Check sheet for the modelled part. Datum: model origin and axes. Units: mm. Face numbers are marked on the shaded views. A direction names the side the tool comes from. Round coordinates to 2 decimals unless told otherwise and drop trailing zeros. Loops run counter-clockwise (first coordinate to the right, second up) from the corner with the lowest first, then second, coordinate; pieces in that order, holes last. Notation, with made-up numbers: M 87,86 L 108,86 A23 cw 108,95 Z; hole C 64.25,-13 d4. An arc over 180 degrees is marked long. One line per question, with ' | ' between items. Start each with the question number.
(1) Section check A-A (x = 0). Record the boundary of the cut face in (y, z), and give its area (3 significant figures).
(2) Thickness scan on probe 1 along Y at (x, z) = (-45, -3); probe 2 along Y at (x, z) = (-38, -2.5); probe 3 along Y at (x, z) = (0, -1.5). Record the ranges inside material, lowest first. Write a range as [from, to].
(3) Section check C-C (y = 14.5). Record the boundary of the cut face in (x, z), and give its area (3 significant figures).
(4) Section check D-D (z = 0). Count the separate pieces of the cut face and the enclosed holes in it, and give its area (3 significant figures).
(5) Draft check along X on the marked faces 4, 5 and 6. Enter one of: +X half, -X half, draft (parallel to the pull), parting line (faces both ways), or undercut.
(6) Tool access check on the marked faces 1, 2 and 3. Record the directions out of +Z, -Z, +X, -X, +Y, -Y that give a thin tool (end or side, any length) a straight path to the whole face; none if there is none.
(7) Section check B-B (x = -39). Record the boundary of the cut face in (y, z), and give its area (3 significant figures).
(8) Go/stop test with flat-tipped pins: P1, Ø1.6, axis at y = 5.5, z = -1, coming from the +X side; P2, Ø4, axis at x = -44.5, z = 2, coming from the +Y side; P3, Ø1.5, axis at x = -20.5, y = 3.5, coming from the -Z side; P4, Ø3.5, axis at y = -40, z = 1, coming from the +X side. Record where each tip stops, or that it passes through.
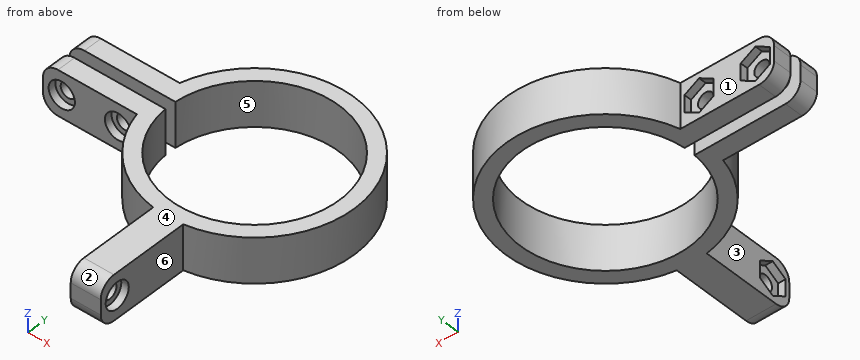
```python
from build123d import *

# Parameters (mm, degrees)
F1_DEPTH  = 6
F6_DEPTH  = 2
F7_DEPTH  = 2
F2_R      = 2.05
F8_DEPTH  = 13
F2_R_2    = 3.5
F9_DEPTH  = 2
F4_R      = 2.05
F10_DEPTH = 8
F4_R_2    = 3.5
F11_DEPTH = 2
F12_R     = 4


with BuildPart() as f1:
    # F0 (on Top) → F1 (new body, symmetric)
    with BuildSketch(Plane.XY):
        with BuildLine():
            ThreePointArc((-22.449944, 1.5), (22.5, 0), (-22.449944, -1.5))
            Line((-22.449944, -1.5), (-50.690465, -1.5))
            Line((-50.690465, -1.5), (-50.690465, -6.5))
            Line((-50.690465, -6.5), (-25.690465, -6.5))
            ThreePointArc((-25.690465, -6.5), (-17.814817, -19.618417), (-4, -26.196374))
            Line((-4, -26.196374), (-4, -51.196374))
            Line((-4, -51.196374), (4, -51.196374))
            Line((4, -51.196374), (4, -26.196374))
            ThreePointArc((4, -26.196374), (19.618417, 17.814817), (-25.690465, 6.5))
            Line((-25.690465, 6.5), (-50.690465, 6.5))
            Line((-50.690465, 6.5), (-50.690465, 1.5))
            Line((-50.690465, 1.5), (-22.449944, 1.5))
        make_face()
    extrude(amount=F1_DEPTH, both=True)

    # F5 (on face) → F6 (cut)
    with BuildSketch(Plane(origin=(-4, 0, 0), x_dir=(0, -1, 0), z_dir=(-1, 0, 0))):
        Polygon((50.093488, -2.25), (50.093488, 2.25), (46.196374, 4.5), (42.299259, 2.25), (42.299259, -2.25), (46.196374, -4.5), align=None)
    extrude(amount=-F6_DEPTH, mode=Mode.SUBTRACT)

    # F3 (on face) → F7 (cut)
    with BuildSketch(Plane(origin=(0, 6.5, 0), x_dir=(-1, 0, 0), z_dir=(0, 1, 0))):
        Polygon((49.587579, -2.25), (49.587579, 2.25), (45.690465, 4.5), (41.793351, 2.25), (41.793351, -2.25), (45.690465, -4.5), align=None)
        Polygon((34.587579, 2.25), (30.690465, 4.5), (26.793351, 2.25), (26.793351, -2.25), (30.690465, -4.5), (34.587579, -2.25), align=None)
    extrude(amount=-F7_DEPTH, mode=Mode.SUBTRACT)

    # F2 (on face) → F8 (cut, through all)
    with BuildSketch(Plane.XZ.offset(6.5)):
        with Locations((-45.690465, 0)):
            Circle(F2_R)
        with Locations((-30.690465, 0)):
            Circle(F2_R)
    extrude(amount=-F8_DEPTH, mode=Mode.SUBTRACT)

    # F2 (on face) → F9 (cut)
    with BuildSketch(Plane.XZ.offset(6.5)):
        with Locations((-45.690465, 0)):
            Circle(F2_R_2)
        with Locations((-45.690465, 0)):
            Circle(F2_R, mode=Mode.SUBTRACT)
        with Locations((-30.690465, 0)):
            Circle(F2_R_2)
        with Locations((-30.690465, 0)):
            Circle(F2_R, mode=Mode.SUBTRACT)
    extrude(amount=-F9_DEPTH, mode=Mode.SUBTRACT)

    # F4 (on face) → F10 (cut, through all)
    with BuildSketch(Plane.YZ.offset(4)):
        with Locations((-46.196374, 0)):
            Circle(F4_R)
    extrude(amount=-F10_DEPTH, mode=Mode.SUBTRACT)

    # F4 (on face) → F11 (cut)
    with BuildSketch(Plane.YZ.offset(4)):
        with Locations((-46.196374, 0)):
            Circle(F4_R_2)
        with Locations((-46.196374, 0)):
            Circle(F4_R, mode=Mode.SUBTRACT)
    extrude(amount=-F11_DEPTH, mode=Mode.SUBTRACT)

    # F12
    f12_edges = [f1.edges().sort_by_distance(p)[0] for p in [
        (-50.690465, 4, 6),
        (-50.690465, 4, -6),
        (-50.690465, -4, 6),
        (-50.690465, -4, -6),
        (0, -51.196374, 6),
        (0, -51.196374, -6),
    ]]
    fillet(f12_edges, radius=F12_R)


solid = f1.part
```
The answers:
1) outline: M -51.2,-2 A4 ccw -47.2,-6 L -22.5,-6 L -22.5,6 L -47.2,6 A4 ccw -51.2,2 Z; M 22.5,-6 L 26.5,-6 L 26.5,6 L 22.5,6 Z; hole C -46.2,0 d4.1 | area: 372 mm²
2) probe 1: [-4.5, -1.5], [1.5, 4.5] | probe 2: [-6.5, -1.5], [1.5, 6.5] | probe 3: [-51.2, -47.59], [-44.8, -22.5], [22.5, 26.5]
3) outline: M -22.18,-6 L -17.2,-6 L -17.2,6 L -22.18,6 Z; M 17.2,-6 L 22.18,-6 L 22.18,6 L 17.2,6 Z | area: 119 mm²
4) separate pieces: 6 | enclosed holes: 0 | area: 893 mm²
5) face 4: draft | face 5: undercut | face 6: +X half
6) face 1: +Z, -Z, -X, +Y | face 2: +Z, +X, -X, -Y | face 3: +Z, -Z, -X, -Y
7) outline: M -6.5,-6 L -1.5,-6 L -1.5,6 L -6.5,6 Z; M 1.5,-6 L 6.5,-6 L 6.5,6 L 1.5,6 Z | area: 120 mm²
8) P1: x = 26.08 | P2: y = 6.5 | P3: through | P4: x = 4
